Here's how the part is built. I have some questions about the finished solid (model axes, mm). Face numbers are marked on the shaded views. A direction names the side the tool comes from. Round coordinates to 2 decimals unless told otherwise and drop trailing zeros. Write each loop counter-clockwise with the first axis right and the second up, starting at its lowest first coordinate (ties: lowest second). Pieces come first, ordered by that corner, then holes. Notation, with made-up numbers: M 80,52 L 132,52 A23 ccw 132,81 Z; hole C 78,1 d1. An arc over 180 degrees is marked long. Use one line per item in the form item = value. Start each with the question number.
Q1. We'd pull the mould along X, two halves only. Please class the marked faces 1, 2 and 3: +X half, -X half, draft (parallel to the pull), parting line (faces both ways), or undercut.
Q2. For the marked faces 4 and 5, which set-ups out of +Z, -Z, +X, -X, +Y, -Y let a thin tool reach every point of the face, with its end or its side?
Q3. I want a section at C-C on z = 10.25. List the corners of the cut face in (x, y) for me.
Q4. I'm going to push flat-ended pins straight in: pin 1 Ø1.1 at (y, z) = (1.5, 0.5) entering from -X; pin 2 Ø1.1 at (y, z) = (-1.5, 0.5) entering from +X; pin 3 Ø0.5 at (x, y) = (0, -2) entering from -Z. Where does each tip first touch, or does it pass through?
Q5. I want a section at A-A on y = 0. List the corners of the cut face in (x, z) for me, and give its area (3 significant figures).
Q6. I want a section at B-B on x = 0. List the corners of the cut face in (y, z) for me, and give its area (3 significant figures).
Q7. I need wall thicknesses on line 1 along Y through (x, z) = (0, 1.8); line 2 along X through (y, z) = (1.1, 4.25) (3 decimals); line 3 along Z through (x, y) = (-0.2, 0.1). Which ranges of each line are inside material? Lowest first, please. Write a range as from..to.
Q8. I want a section at D-D on z = 8.5. List the corners of the cut face in (x, y) for me.
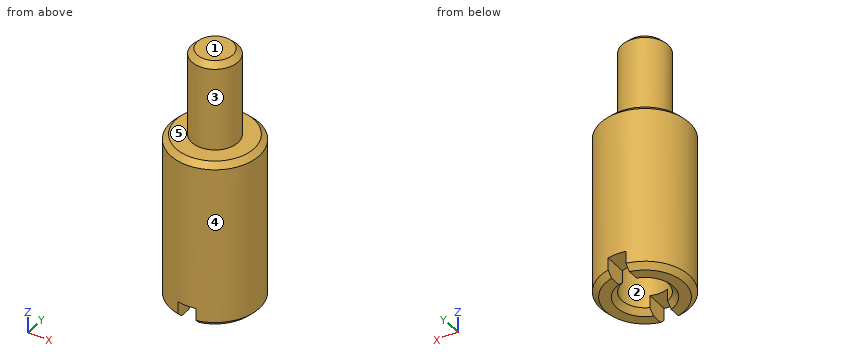
Autodesk Inventor part; units mm, degrees
ref_plane "YZ Plane" through (0, 0, 0) normal (1, 0, 0) x (0, 1, 0)
ref_plane "XZ Plane" through (0, 0, 0) normal (0, 1, 0) x (-1, 0, 0)
ref_plane "XY Plane" through (0, 0, 0) normal (0, 0, 1) x (1, 0, 0)
sketch "スケッチ1" plane through (0, 0, 0) normal (0, 1, 0) x (-1, 0, 0)
  line L0 (-1.6, 0) -> (-2.2, 0)
  line L1 (-2.5, 0.3) -> (-2.5, 9.2)
  line L2 (-2.2, 9.5) -> (-1.3, 9.5)
  line L3 (-1.3, 9.5) -> (-1.3, 14.2)
  line L4 (-1, 14.5) -> (0, 14.5)
  line L5 (0, 14.5) -> (0, 5)
  line L6 (0, 5) -> (-1.3, 5)
  line L7 (-1.3, 5) -> (-1.3, 0.3)
  line L8 (-1.3, 14.2) -> (-1, 14.5)
  line L9 (-2.5, 9.2) -> (-2.2, 9.5)
  line L10 (-2.5, 0.3) -> (-2.2, 0)
  line L11 (-1.6, 0) -> (-1.3, 0.3)
  line L12 (0, -2.9) -> (0, 17.4)
  point P0 (0, 0)
  point P1 (-2.5, 0)
  point P2 (-2.5, 9.5)
  point P3 (-1.3, 14.5)
  point P4 (-1.3, 0)
  dimension "d0" = 2.6
  dimension "d1" = 5
  dimension "d2" = 9.5
  dimension "d3" = 5
  dimension "d4" = 5
  dimension "d5" = 2.6
  dimension "d6" = 0.3
  dimension "d7" = 0.3
  dimension "d8" = 0.3
  dimension "d9" = 0.3
  dimension "d10" = 0.3
  dimension "d11" = 0.3
  dimension "d12" = 0.3
  dimension "d13" = 0.3
revolve "回転1" add sketch "スケッチ1" angle 360 about axis through (0, 0, -10) along (0, 0, 1)
thread "ねじ1"
thread "ねじ2"
sketch "スケッチ2" plane through (0, 0, 0) normal (0, 0, -1) x (-1, 0, 0)
  line L0 (-0.5, 2.5) -> (0.5, 2.5)
  line L1 (0.5, 2.5) -> (0.5, -2.5)
  line L2 (0.5, -2.5) -> (-0.5, -2.5)
  line L3 (-0.5, -2.5) -> (-0.5, 2.5)
  line L4 (-0.5, 2.5) -> (0.5, -2.5) construction
  line L5 (0.5, 2.5) -> (-0.5, -2.5) construction
  circle A0 centre (0, 0) radius 2.5
  point P0 (0.5, 2.4495)
  point P1 (-0.5, 2.4495)
  point P2 (-0.5, -2.4495)
  point P3 (0.5, -2.4495)
  dimension "d19" = 1
extrude "押し出し1" cut sketch "スケッチ2" against normal blind 1 contours A0 L1 L3
properties part number "BRU-2609.5S" material "ステンレス鋼 AISI 304"
Reported:
q1.face_1 = draft
q1.face_2 = undercut
q1.face_3 = parting line
q2.face_4 = +Z, -Z
q2.face_5 = +Z
q3.outline = C 0,0 d2.6
q4.pin_1 = -2.31
q4.pin_2 = 2.31
q4.pin_3 = 1
q5.outline = M -2.5,0.3 L -2.2,0 L -1.6,0 L -1.3,0.3 L -1.3,5 L 1.3,5 L 1.3,0.3 L 1.6,0 L 2.2,0 L 2.5,0.3 L 2.5,9.2 L 2.2,9.5 L 1.3,9.5 L 1.3,14.2 L 1,14.5 L -1,14.5 L -1.3,14.2 L -1.3,9.5 L -2.2,9.5 L -2.5,9.2 Z
q5.area = 47.1 mm^2
q6.outline = M -2.5,1 L -1.3,1 L -1.3,5 L 1.3,5 L 1.3,1 L 2.5,1 L 2.5,9.2 L 2.2,9.5 L 1.3,9.5 L 1.3,14.2 L 1,14.5 L -1,14.5 L -1.3,14.2 L -1.3,9.5 L -2.2,9.5 L -2.5,9.2 Z
q6.area = 44.9 mm^2
q7.line_1 = -2.5..-1.3, 1.3..2.5
q7.line_2 = -2.245..-0.693, 0.693..2.245
q7.line_3 = 5..14.5
q8.outline = C 0,0 d5
